Here's how the part is built. I have some questions about the finished solid (model axes, mm). A direction names the side the tool comes from. Coordinates: 2 decimals unless noted, no trailing zeros. Order: outer loops, then holes, each group sorted by start corner. A loop starts at its lowest first (then second) coordinate and runs counter-clockwise, first axis right, second up. Notation, with made-up numbers: (6, 76) - (56, 76) arc R19 ccw to (56, 86) - close; hole circle Ø9 at (6.25, 60). An arc over 180 degrees is marked (long way). Answer in a Markdown table with one row per item. Add a question column.
Item 1: On a 3-axis mill with a long thin cutter (end or side, diameter ignored), from which of +Z, -Z, +X, -X, +Y, -Y can I reach the whole of each face in a straight line? I mean faces 5 (the flat face through (-128.875, 36, 0)), 6 (the flat face through (18, 11.4, 0)), 7 (the flat face through (-15, 14, 0)). Say none if no direction works.
Item 2: Will these pins go through, and if not, where does the flat tip stop? pin 1 Ø18 at (x, z) = (-58, 0) entering from -Y; pin 2 Ø15 at (x, y) = (-84.5, 34) entering from +Z; pin 3 Ø5 at (y, z) = (16.5, 25.5) entering from +X (3 decimals).
Item 3: I want a section at B-B (z = 43.5). Please give me the cut outline in (x, y) (3 decimals).
Item 4: I want a section at A-A (x = -114.5). Please give me the cut outline in (y, z).
Item 5: Thinking about a two-plate mould opening in Y: for faces 1 (the flat face through (-53, 36, -14.8)), 2 (the flat face through (-53, 36, 14.8)), 3 (the flat face through (-156, 36, 56.145)), 4 (the flat face through (-18, 5, -15)), which applies, +Y half, -Y half, draft (parallel to the pull), parting line (faces both ways), or undercut?
Item 6: If I drill on line 1 along Y through (x, z) = (18.5, -8.5); line 2 along Z through (x, y) = (-88.5, 22); line 3 along Y through (x, z) = (-128, -7), over which ranges is the centre line in solid material (lowest first)? Write a range as from..to.
```python
from build123d import *

# Parameters (mm, degrees)
SKETCH1_W                = 42.25
SKETCH1_H                = 35.6
BOSS_EXTRUDE1_DEPTH      = 2
SKETCH2_W                = 2
SKETCH2_H                = 35.6
BOSS_EXTRUDE2_DEPTH      = 50
SKETCH1_2_W              = 42.25
SKETCH1_2_H              = 35.6
CUT_EXTRUDE6_DEPTH       = 20
SKETCH8_W                = 42.25
SKETCH8_H                = 35.6
BOSS_EXTRUDE3_DEPTH      = 2
SKETCH9_W                = 35.6
SKETCH9_H                = 13
BOSS_EXTRUDE4_DEPTH      = 42.25
SKETCH12_W               = 30
SKETCH12_H               = 13
CUT_EXTRUDE9_DEPTH       = 36.6
SKETCH13_W               = 24.4
SKETCH13_H               = 13
CUT_EXTRUDE10_DEPTH      = 37.125
CUT_EXTRUDE10_DEPTH_BACK = 7.125
SKETCH15_R               = 1.35
CUT_EXTRUDE11_DEPTH      = 43.25
SKETCH16_W               = 35.6
SKETCH16_H               = 35.754688938
BOSS_EXTRUDE5_DEPTH      = 150
SKETCH18_W               = 112.087725711
SKETCH18_H               = 105.02156137
BOSS_EXTRUDE6_DEPTH      = 5
SKETCH20_W               = 72.087725711
SKETCH20_H               = 65.02156137
SKETCH17_W               = 52.087725711
SKETCH17_H               = 45.02156137
SKETCH21_W               = 29.6
SKETCH21_H               = 29.754688938
CUT_EXTRUDE13_DEPTH      = 150
SKETCH25_W               = 24.4
SKETCH25_H               = 6.6
BOSS_EXTRUDE9_DEPTH      = 6.125
SKETCH26_W               = 24.4
SKETCH26_H               = 6.6
BOSS_EXTRUDE10_DEPTH     = 6.125
SKETCH27_R               = 1.35
CUT_EXTRUDE15_DEPTH      = 42.25


with BuildPart() as part:
    # Sketch1 → Boss-Extrude1 (new body)
    with BuildSketch(Plane(origin=(0, 0, 0), x_dir=(1, 0, 0), z_dir=(0, 1, 0))):
        Rectangle(SKETCH1_W, SKETCH1_H)
    extrude(amount=BOSS_EXTRUDE1_DEPTH)

    # Sketch2 → Boss-Extrude2 (add)
    with BuildSketch(Plane(origin=(0, 2, 0), x_dir=(1, 0, 0), z_dir=(0, 1, 0))):
        with Locations((-20.125, 0)):
            Rectangle(SKETCH2_W, SKETCH2_H)
        with Locations((20.125, 0)):
            Rectangle(SKETCH2_W, SKETCH2_H)
    extrude(amount=BOSS_EXTRUDE2_DEPTH)

    # Sketch1<2> → Cut-Extrude6 (cut)
    with BuildSketch(Plane(origin=(0, 0, 0), x_dir=(1, 0, 0), z_dir=(0, 1, 0))):
        Rectangle(SKETCH1_2_W, SKETCH1_2_H)
    extrude(amount=CUT_EXTRUDE6_DEPTH, mode=Mode.SUBTRACT)

    # Sketch8 → Boss-Extrude3 (add)
    with BuildSketch(Plane.XZ.offset(-20)):
        Rectangle(SKETCH8_W, SKETCH8_H)
    extrude(amount=BOSS_EXTRUDE3_DEPTH)

    # Sketch9 → Boss-Extrude4 (add)
    with BuildSketch(Plane(origin=(21.125, 0, 0), x_dir=(0, 0, -1), z_dir=(1, 0, 0))):
        with Locations((0, 11.5)):
            Rectangle(SKETCH9_W, SKETCH9_H)
    extrude(amount=-BOSS_EXTRUDE4_DEPTH)

    # Sketch12 → Cut-Extrude9 (cut, through all)
    with BuildSketch(Plane(origin=(0, 0, -17.8), x_dir=(-1, 0, 0), z_dir=(0, 0, -1))):
        with Locations((0, 11.5)):
            Rectangle(SKETCH12_W, SKETCH12_H)
    extrude(amount=-CUT_EXTRUDE9_DEPTH, mode=Mode.SUBTRACT)

    # Sketch13 → Cut-Extrude10 (cut, two sides)
    with BuildSketch(Plane.ZY.offset(-15)) as cut_extrude10_sk:
        with Locations((0, 11.5)):
            Rectangle(SKETCH13_W, SKETCH13_H)
    extrude(amount=CUT_EXTRUDE10_DEPTH, mode=Mode.SUBTRACT)
    extrude(cut_extrude10_sk.sketch, amount=-CUT_EXTRUDE10_DEPTH_BACK, mode=Mode.SUBTRACT)

    # Sketch15 → Cut-Extrude11 (cut, through all)
    with BuildSketch(Plane.ZY.offset(21.125)):
        with Locations((-15, 7.9)):
            Circle(SKETCH15_R)
        with Locations((15, 7.9)):
            Circle(SKETCH15_R)
    extrude(amount=-CUT_EXTRUDE11_DEPTH, mode=Mode.SUBTRACT)

    # Sketch16 → Boss-Extrude5 (add)
    with BuildSketch(Plane(origin=(21.125, 0, 0), x_dir=(0, 0, -1), z_dir=(1, 0, 0))):
        with Locations((0, 35.877344469)):
            Rectangle(SKETCH16_W, SKETCH16_H)
    extrude(amount=-BOSS_EXTRUDE5_DEPTH)



with BuildPart() as body_2:
    # Sketch18 → Boss-Extrude6 (new body)
    with BuildSketch(Plane.ZY.offset(158.875)):
        with Locations((0.100945205, 36.893036207)):
            Rectangle(SKETCH18_W, SKETCH18_H)
    extrude(amount=-BOSS_EXTRUDE6_DEPTH)


with BuildPart() as part_1:
    add(part.part)

    add(body_2.part)  # Loft1 merges body 2
    # Sketch20 → Loft1 section 0
    with BuildSketch(Plane(origin=(-153.875, 0, 0), x_dir=(0, 0, -1), z_dir=(1, 0, 0))):
        with Locations((-0.100945205, 36.893036207)):
            Rectangle(SKETCH20_W, SKETCH20_H)
    # Sketch17 → Loft1 section 1
    with BuildSketch(Plane.ZY.offset(128.875)):
        with Locations((0.100945205, 36.893036207)):
            Rectangle(SKETCH17_W, SKETCH17_H)
    loft()

    # Sketch21 → Cut-Extrude13 (cut)
    with BuildSketch(Plane(origin=(21.125, 0, 0), x_dir=(0, 0, -1), z_dir=(1, 0, 0))):
        with Locations((0, 35.877344469)):
            Rectangle(SKETCH21_W, SKETCH21_H)
    extrude(amount=-CUT_EXTRUDE13_DEPTH, mode=Mode.SUBTRACT)

    # Sketch25 → Boss-Extrude9 (add)
    with BuildSketch(Plane(origin=(21.125, 0, 0), x_dir=(0, 0, -1), z_dir=(1, 0, 0))):
        with Locations((0, 14.7)):
            Rectangle(SKETCH25_W, SKETCH25_H)
    extrude(amount=-BOSS_EXTRUDE9_DEPTH)

    # Sketch26 → Boss-Extrude10 (add)
    with BuildSketch(Plane(origin=(-15, 0, 0), x_dir=(0, 0, -1), z_dir=(1, 0, 0))):
        with Locations((0, 14.7)):
            Rectangle(SKETCH26_W, SKETCH26_H)
    extrude(amount=-BOSS_EXTRUDE10_DEPTH)

    # Sketch27 → Cut-Extrude15 (cut)
    with BuildSketch(Plane(origin=(21.125, 0, 0), x_dir=(0, 0, -1), z_dir=(1, 0, 0))):
        with Locations((8.5, 14.2)):
            Circle(SKETCH27_R)
        with Locations((-8.5, 14.2)):
            Circle(SKETCH27_R)
    extrude(amount=-CUT_EXTRUDE15_DEPTH, mode=Mode.SUBTRACT)


solid = part_1.part
```
Values follow:
| question | item | result |
|---|---|---|
| 1 | face 5 | +X |
| 1 | face 6 | +X, -Y |
| 1 | face 7 | +Z, -Z, -Y |
| 2 | pin 1 | stops at y = 18 |
| 2 | pin 2 | stops at z = 17.8 |
| 2 | pin 3 | stops at x = -128.875 |
| 3 | outline | (-158.875, -15.618) - (-153.875, -15.618) - (-153.875, 89.404) - (-158.875, 89.404) - close |
| 4 | outline | (18, -17.8) - (53.75, -17.8) - (53.75, 17.8) - (18, 17.8) - close; hole (21, -14.8) - (50.75, -14.8) - (50.75, 14.8) - (21, 14.8) - close |
| 5 | face 1 | undercut |
| 5 | face 2 | undercut |
| 5 | face 3 | draft |
| 5 | face 4 | -Y half |
| 6 | line 1 | y = 11.4..12.85, 15.55..21, 50.75..53.75 |
| 6 | line 2 | z = -17.8..-14.8, 14.8..17.8 |
| 6 | line 3 | y = 18..21, 50.75..53.75 |
